from build123d import *

# Parameters (mm, degrees)
SKETCH1_W           = 10
SKETCH1_H           = 100
BOSS_EXTRUDE1_DEPTH = 4
CUT_EXTRUDE1_DEPTH  = 4
CHAMFER1_SIZE       = 5
SKETCH3_R           = 2
BOSS_EXTRUDE2_DEPTH = 10


with BuildPart() as part:
    # Sketch1 → Boss-Extrude1 (new body)
    with BuildSketch(Plane.XY):
        Rectangle(SKETCH1_W, SKETCH1_H)
    extrude(amount=BOSS_EXTRUDE1_DEPTH)

    # Sketch2 → Cut-Extrude1 (cut)
    with BuildSketch(Plane.XY.offset(4)):
        Polygon((5, 50), (-5, 35.718519933), (-5, 50), align=None)
    extrude(amount=-CUT_EXTRUDE1_DEPTH, mode=Mode.SUBTRACT)

    # Chamfer1
    chamfer1_edges = [part.edges().sort_by_distance(p)[0] for p in [
        (-5, -50, 2),
        (5, -50, 2),
    ]]
    chamfer(chamfer1_edges, length=CHAMFER1_SIZE - 0.0001)  # a hair under: the kernel refuses the full size

    # Sketch3 → Boss-Extrude2 (add)
    with BuildSketch(Plane.XY.offset(4)):
        with Locations((0, 34)):
            Circle(SKETCH3_R)
    extrude(amount=-BOSS_EXTRUDE2_DEPTH)


solid = part.part
Geometry: final body of the model. Coordinates: model frame, mm. A direction names the side the tool comes from. Give positions to 0.01 mm unless a question says otherwise; leave off trailing zeros. Order: outer loops, then holes, each group sorted by start corner. A loop starts at its lowest first (then second) coordinate and runs counter-clockwise, first axis right, second up. Notation, with made-up numbers: (71, 86) -> (78, 86) arc R19 cw to (78, 108) -> close; hole circle Ø5 at (-4, 57.25). An arc over 180 degrees is marked (long way). Answer as a JSON object with one key per item and string values.
Q1. Section B-B (z = -4). Output: boundary loops of the cut face in (x, y).
Entries:
{"outline": "circle Ø4 at (0, 34)"}
Q2. First-contact query: pin 1 (3 mm diameter, centred on x = 3.5, y = 4, fed in from -Z); pin 2 (2 mm diameter, centred on x = -4, z = -4.5, fed in from +Y); pin 3 (1.5 mm diameter, centred on x = -0.5, z = -3, fed in from -Y). Flat tips, straight axial feed; report the tip coordinate or a pass-through.
Entries:
{"pin 1": "stops at z = 0", "pin 2": "passes through", "pin 3": "stops at y = 32"}
Q3. Access query for faces 1 (the flat face through (0, 1, 4)), 2 (the cylindrical face through (0, 32, -3)). Directions: +Z, -Z, +X, -X, +Y, -Y. A direction counts if a zero-diameter tool reaches every point of the face in a straight line with its end or side. Return the directions, or none.
Entries:
{"face 1": "+Z, +X, -X, +Y, -Y", "face 2": "-Z"}
Q4. Section C-C (x = 3). Output: boundary loops of the cut face in (y, z).
Entries:
{"outline": "(-47, 0) -> (47.14, 0) -> (47.14, 4) -> (-47, 4) -> close"}
Q5. Section A-A (y = 34). Output: boundary loops of the cut face in (x, z), plus the area to 3 significant figures.
Entries:
{"outline": "(-5, 0) -> (-2, 0) -> (-2, -6) -> (2, -6) -> (2, 0) -> (5, 0) -> (5, 4) -> (-5, 4) -> close", "area": "64.0 mm^2"}
Q6. Section D-D (y = -30.5). Output: boundary loops of the cut face in (x, z), plus the area to 3 significant figures.
Entries:
{"outline": "(-5, 0) -> (5, 0) -> (5, 4) -> (-5, 4) -> close", "area": "40.0 mm^2"}
Q7. Material intervals for probe 1 along Z at (x, y) = (-3.5, -45); probe 2 along Y at (x, z) = (0, -2.75); probe 3 along Y at (x, z) = (0.5, -5.25), sorted ascending.
Entries:
{"probe 1": "z = 0 to 4", "probe 2": "y = 32 to 36", "probe 3": "y = 32.06 to 35.94"}
